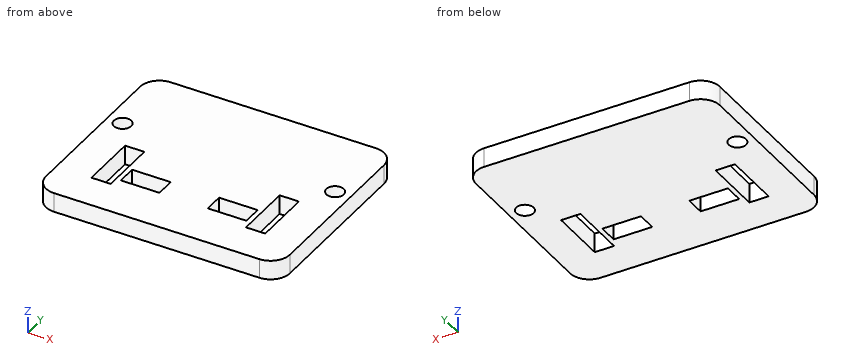
```python
from build123d import *

# Parameters (mm, degrees)
SKETCH1_R                      = 11.422
BOSS_EXTRUDE1_DEPTH            = 25.4
SKETCH2_W                      = 50.8
SKETCH2_H                      = 25.4
FOAM_INSERT_CUT_THROUGHS_DEPTH = 25.4
SKETCH3_W                      = 25.4
SKETCH3_H                      = 76.2
CUT_EXTRUDE1_DEPTH             = 25.4


with BuildPart() as part:
    # Sketch1 → Boss-Extrude1 (new body)
    with BuildSketch(Plane.XY):
        with BuildLine():
            Line((-134.937453137, -131.801904544), (134.937453137, -131.801904544))
            ThreePointArc((134.937453137, -131.801904544), (152.897965379, -124.362416786), (160.337453137, -106.401904544))
            Line((160.337453137, -106.401904544), (160.337453137, 106.401904544))
            ThreePointArc((160.337453137, 106.401904544), (152.897965379, 124.362416786), (134.937453137, 131.801904544))
            Line((134.937453137, 131.801904544), (-134.937453137, 131.801904544))
            ThreePointArc((-134.937453137, 131.801904544), (-152.897965379, 124.362416786), (-160.337453137, 106.401904544))
            Line((-160.337453137, 106.401904544), (-160.337453137, -106.401904544))
            ThreePointArc((-160.337453137, -106.401904544), (-152.897965379, -124.362416786), (-134.937453137, -131.801904544))
        make_face()
        with Locations((-139.7, 31.289898812)):
            Circle(SKETCH1_R, mode=Mode.SUBTRACT)
        with Locations((139.7, 31.289898812)):
            Circle(SKETCH1_R, mode=Mode.SUBTRACT)
    extrude(amount=BOSS_EXTRUDE1_DEPTH)

    # Sketch2 → Foam Insert Cut-Throughs (cut)
    with BuildSketch(Plane(origin=(0, 0, 0), x_dir=(-1, 0, 0), z_dir=(0, 0, -1))):
        with Locations((-57.15, -58.30002437)):
            Rectangle(SKETCH2_W, SKETCH2_H)
        with Locations((57.15, -58.30002437)):
            Rectangle(SKETCH2_W, SKETCH2_H)
    extrude(amount=-FOAM_INSERT_CUT_THROUGHS_DEPTH, mode=Mode.SUBTRACT)

    # Sketch3 (on Front Plane) → Cut-Extrude1 (cut)
    with BuildSketch(Plane.XY):
        with Locations((-101.6, -44.910101188)):
            Rectangle(SKETCH3_W, SKETCH3_H)
        with Locations((101.6, -44.910101188)):
            Rectangle(SKETCH3_W, SKETCH3_H)
    extrude(amount=CUT_EXTRUDE1_DEPTH, mode=Mode.SUBTRACT)


solid = part.part
```
Part model, mm, in its own coordinate system. Give positions to 0.01 mm unless a question says otherwise; leave off trailing zeros. Order: outer loops, then holes, each group sorted by start corner. A loop starts at its lowest first (then second) coordinate and runs counter-clockwise, first axis right, second up. Notation, with made-up numbers: (48, 57.25) - (87, 57.25) arc R29 ccw to (87, 92.25) - close; hole circle Ø3 at (-13.5, 87.25). An arc over 180 degrees is marked (long way). Use one line per item in the form item = value.
Item 1: Probe probe 1 along X at (y, z) = (-19, 5.25); probe 2 along X at (y, z) = (30.5, 7.25); probe 3 along X at (y, z) = (-51, 5.25). List the from-to ranges inside material, lowest first. Write a range as from..to.
Solution:
probe_1 = -160.34..-114.3, -88.9..88.9, 114.3..160.34
probe_2 = -160.34..-151.09, -128.31..128.31, 151.09..160.34
probe_3 = -160.34..-114.3, -88.9..-82.55, -31.75..31.75, 82.55..88.9, 114.3..160.34
Item 2: Slice it at C-C on y = -17. Give the cut face in (x, z), and give its area (3 significant figures).
Solution:
outline = (-160.34, 0) - (-114.3, 0) - (-114.3, 25.4) - (-160.34, 25.4) - close; (-88.9, 0) - (88.9, 0) - (88.9, 25.4) - (-88.9, 25.4) - close; (114.3, 0) - (160.34, 0) - (160.34, 25.4) - (114.3, 25.4) - close
area = 6,850 mm2
Item 3: Slice it at B-B on y = -63. Give the cut face in (x, z), and give its area (3 significant figures).
Solution:
outline = (-160.34, 0) - (-114.3, 0) - (-114.3, 25.4) - (-160.34, 25.4) - close; (-88.9, 0) - (-82.55, 0) - (-82.55, 25.4) - (-88.9, 25.4) - close; (-31.75, 0) - (31.75, 0) - (31.75, 25.4) - (-31.75, 25.4) - close; (82.55, 0) - (88.9, 0) - (88.9, 25.4) - (82.55, 25.4) - close; (114.3, 0) - (160.34, 0) - (160.34, 25.4) - (114.3, 25.4) - close
area = 4,270 mm2
Item 4: Slice it at A-A on x = -108. Give the cut face in (y, z).
Solution:
outline = (-131.8, 0) - (-83.01, 0) - (-83.01, 25.4) - (-131.8, 25.4) - close; (-6.81, 0) - (131.8, 0) - (131.8, 25.4) - (-6.81, 25.4) - close
Item 5: Slice it at D-D on z = 4.5. Give the cut face in (x, y), and give its area (3 significant figures).
Solution:
outline = (-160.34, -106.4) arc R25.4 ccw to (-134.94, -131.8) - (134.94, -131.8) arc R25.4 ccw to (160.34, -106.4) - (160.34, 106.4) arc R25.4 ccw to (134.94, 131.8) - (-134.94, 131.8) arc R25.4 ccw to (-160.34, 106.4) - close; hole circle Ø22.84 at (-139.7, 31.29); hole (-114.3, -83.01) - (-88.9, -83.01) - (-88.9, -6.81) - (-114.3, -6.81) - close; hole (-82.55, -71) - (-31.75, -71) - (-31.75, -45.6) - (-82.55, -45.6) - close; hole (31.75, -71) - (82.55, -71) - (82.55, -45.6) - (31.75, -45.6) - close; hole (88.9, -83.01) - (114.3, -83.01) - (114.3, -6.81) - (88.9, -6.81) - close; hole circle Ø22.84 at (139.7, 31.29)
area = 76,700 mm2
